```python
from build123d import *

# Parameters (mm, degrees)
SKETCH1_W                   = 35
SKETCH1_H                   = 40
BOSS_EXTRUDE1_DEPTH         = 75
CUT_EXTRUDE1_REACH          = 88.783
FILLET1_R                   = 3
FILLET2_R                   = 5
M6_TAPPED_HOLE1_D           = 5
M6_TAPPED_HOLE1_DEPTH       = 17
M6_TAPPED_HOLE1_CSINK_D     = 6.05
M6_TAPPED_HOLE1_CSINK_ANGLE = 90
M6_TAPPED_HOLE1_TIP         = 1.502151548
FILLET3_R                   = 1


with BuildPart() as part:
    # Sketch1 → Boss-Extrude1 (new body)
    with BuildSketch(Plane(origin=(0, 0, 0), x_dir=(1, 0, 0), z_dir=(0, 1, 0))):
        Rectangle(SKETCH1_W, SKETCH1_H)
    extrude(amount=-BOSS_EXTRUDE1_DEPTH)

    # Sketch2 → Cut-Extrude1 (cut, up to next)
    with BuildSketch(Plane.XY.offset(20), mode=Mode.PRIVATE) as cut_extrude1_sk1:
        with BuildLine():
            Line((-13.631919427, -61.241229517), (-17.5, -59.833363324))
            Line((-17.5, -59.833363324), (-17.5, -75))
            Line((-17.5, -75), (-11, -75))
            Line((-11, -75), (-11, -65))
            ThreePointArc((-11, -65), (-11.723391823, -62.705694255), (-13.631919427, -61.241229517))
        make_face()
    cut_extrude1_tool1 = extrude(cut_extrude1_sk1.sketch, amount=-CUT_EXTRUDE1_REACH, mode=Mode.PRIVATE) & part.part
    add(cut_extrude1_tool1.solids().sort_by_distance((-14.386052, -68.077717, 20))[0], mode=Mode.SUBTRACT)

    # Fillet1
    fillet1_edges = [part.edges().sort_by_distance(p)[0] for p in [
        (-11, -75, 0),
    ]]
    fillet(fillet1_edges, radius=FILLET1_R)

    # Fillet2
    fillet2_edges = [part.edges().sort_by_distance(p)[0] for p in [
        (17.5, -37.5, 20),
        (17.5, -37.5, -20),
    ]]
    fillet(fillet2_edges, radius=FILLET2_R)

    # M6 Tapped Hole1
    with Locations(Plane(origin=(0, 0, 0), x_dir=(1, 0, 0), z_dir=(0, 1, 0))):
        with Locations((0, 12.5), (0, -12.5)):
            CounterSinkHole(M6_TAPPED_HOLE1_D / 2, M6_TAPPED_HOLE1_CSINK_D / 2, depth=M6_TAPPED_HOLE1_DEPTH, counter_sink_angle=M6_TAPPED_HOLE1_CSINK_ANGLE)
            with Locations((0, 0, -(M6_TAPPED_HOLE1_DEPTH + M6_TAPPED_HOLE1_TIP / 2))):  # 118° drill point
                Cone(0, M6_TAPPED_HOLE1_D / 2, M6_TAPPED_HOLE1_TIP, mode=Mode.SUBTRACT)

    # Fillet3
    fillet3_edges = [part.edges().sort_by_distance(p)[0] for p in [
        (-17.5, -29.916681662, -20),
        (-17.5, -29.916681662, 20),
    ]]
    fillet(fillet3_edges, radius=FILLET3_R)


solid = part.part
```
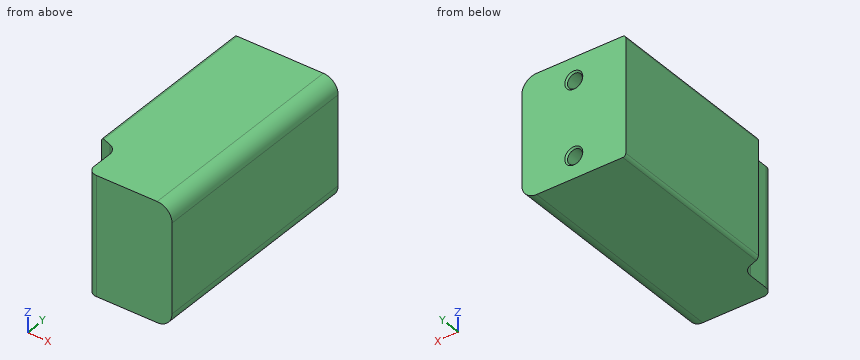
Design review of the part built by this model. Coordinates are the model's own, in mm. Round coordinates to 2 decimals unless told otherwise and drop trailing zeros. Write each loop counter-clockwise with the first axis right and the second up, starting at its lowest first coordinate (ties: lowest second). Pieces come first, ordered by that corner, then holes. Notation, with made-up numbers: (30, 78) -> (57, 78) arc R36 ccw to (57, 112) -> close; hole circle Ø1 at (11.5, -2.5). An arc over 180 degrees is marked (long way). Write item = value, one per line. Start each with the question number.
1) Take a section at A-A, the plane y = -10. State the section outline as (x, z) points, plus the area to 3 significant figures.
2) Clearance check with flat-ended pins moving along their axes: pin 1 (1 mm diameter, centred on x = -11.5, z = 13, fed in from +Y); pin 2 (2 mm diameter, centred on y = -67, z = 1, fed in from -X); pin 3 (4 mm diameter, centred on x = 0, z = 12.5, fed in from +Y). State where each tip first meets the part, or that it passes through.
3) Take a section at B-B, the plane z = -8. State the section outline as (x, y) points.
4) Wall thickness on probe 1 along Z at (x, y) = (0, -4.25); probe 2 along X at (y, z) = (-10, 12.5); probe 3 along X at (y, z) = (-4.5, -10.5): over which ranges is each line inside the solid? List them lowest first. Write a range as from..to.
Results list:
q1.outline = (-17.5, -19) arc R1 ccw to (-16.5, -20) -> (12.5, -20) arc R5 ccw to (17.5, -15) -> (17.5, 15) arc R5 ccw to (12.5, 20) -> (-16.5, 20) arc R1 ccw to (-17.5, 19) -> close; hole circle Ø5 at (0, -12.5); hole circle Ø5 at (0, 12.5)
q1.area = 1,350 mm²
q2.pin_1 = 0
q2.pin_2 = -11
q2.pin_3 = -17.3
q3.outline = (-17.5, -59.83) -> (-13.63, -61.24) arc R4 cw to (-11, -65) -> (-11, -72) arc R3 ccw to (-8, -75) -> (17.5, -75) -> (17.5, 0) -> (-17.5, 0) -> close
q4.probe_1 = -20..-15, -10..10, 15..20
q4.probe_2 = -17.5..-2.5, 2.5..17.5
q4.probe_3 = -17.5..-1.5, 1.5..17.5
